Geometry check sheet. Reference: the model listing, model coordinates, mm. Face numbers are marked on the shaded views. A direction names the side the tool comes from. Round coordinates to 2 decimals unless told otherwise and drop trailing zeros. Order: outer loops, then holes, each group sorted by start corner. A loop starts at its lowest first (then second) coordinate and runs counter-clockwise, first axis right, second up.
(1) Thickness scan on L1, parallel to X at y = -6.5, z = 15.5; L2, parallel to Y at x = -9.5, z = 12; L3, parallel to Y at x = 0.5, z = 14. Record the ranges inside material, lowest first.
(2) Cross-section at C-C on x = 1.5. Enter the section's corners in (y, z).
(3) Set-up check for the marked faces 1, 2 and 3: record each of +Z, -Z, +X, -X, +Y, -Y from which the full face is reachable in a straight line by a thin tool's end or side.
(4) Draft check along X on the marked faces 4, 5, 6 and 7. Enter one of: pulls with the +X half, pulls with the -X half, needs draft (parallel to the pull), parting line crosses it, or undercut.
(5) Gauge pin test, flat ends, axial feed: P1, Ø6, axis at x = -6, y = -4, coming from the -Z side; P2, Ø4, axis at y = -6, z = 25.5, coming from the +X side; P3, Ø16, axis at x = 13, z = 12.5, coming from the +Y side (3 decimals); P4, Ø2, axis at y = 3, z = 18.5, coming from the +X side. Record the tip position at first contact, or that the pin passes through.
(6) Cross-section at B-B on y = -5.5. Enter the section's corners in (x, z).
(7) Cross-section at A-A on z = 15. Count the separate pieces of the cut face and the enclosed holes in it, and give its area (3 significant figures).
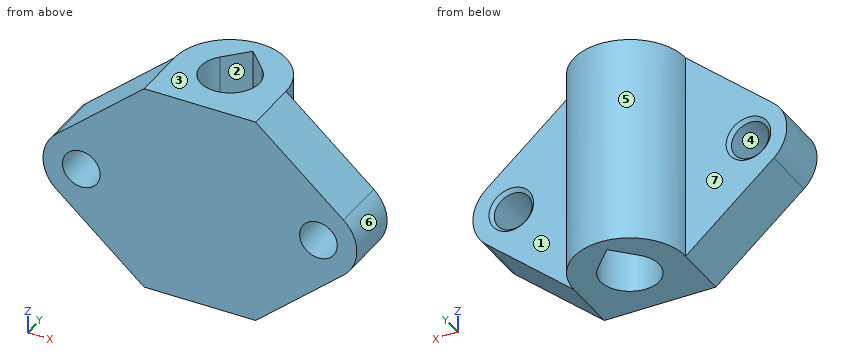
Solid Edge part; units mm, degrees
sketch "Sketch1" plane through (0, 0, 0) normal (0, 0, 1) x (1, 0, 0)
  circle A0 centre (0, 0) radius 4.1
  circle A1 centre (0, 0) radius 8
extrude "Protrusion1" add sketch "Sketch1" along normal blind 30
sketch "Sketch2" plane through (0, -8, 0) normal (0, -1, 0) x (1, 0, 0)
  arc A0 (-20.6265, 10.8649) -> (-20.548, 19.2026) centre (-17, 15) cw
  line L0 (-20.548, 19.2026) -> (-8, 30)
  line L1 (-8, 30) -> (8, 30)
  line L2 (8, 30) -> (20.5873, 19.1691)
  arc A1 (20.5873, 10.8309) -> (20.5873, 19.1691) centre (17, 15) ccw
  line L3 (8, 0) -> (20.5873, 10.8309)
  line L4 (8, 0) -> (-8, 0)
  line L5 (-20.6265, 10.8649) -> (-8, 0)
  circle A2 centre (-17, 15) radius 2.7
  circle A3 centre (17, 15) radius 2.7
extrude "Protrusion2" add sketch "Sketch2" against normal up to vertex (8 mm away)
sketch "Sketch3" plane through (0, 0, 30) normal (0, 0, 1) x (0, 1, 0)
  circle A0 centre (0, 0) radius 4.2
extrude "Cutout1" cut sketch "Sketch3" against normal through all
sketch "Sketch4" plane through (0, 0, 0) normal (0, 0, -1) x (-1, 0, 0)
  line L0 (0, 0) -> (3.0212, 2.9176)
  line L1 (3.0212, 2.9176) -> (0, 6.0461)
  line L2 (0, 6.0461) -> (-3.0212, 2.9176)
  line L3 (-3.0212, 2.9176) -> (0, 0)
extrude "Cutout2" cut sketch "Sketch4" against normal through all
chamfer "Chamfer_1" distance 0.5 angle 45 2 edges at (14.3, 0, 15) (-19.7, 0, 15)
Found:
1. L1: x = -22.48 to -19.65, -14.35 to 14.35, 19.65 to 22.48
1. L2: y = -8 to 0
1. L3: y = -8 to -4.17, 5.53 to 7.98
2. outline: (-8, 0) - (-3.92, 0) - (-3.92, 30) - (-8, 30) - close; (4.49, 0) - (7.86, 0) - (7.86, 30) - (4.49, 30) - close
3. face 1: +Z, -Z, +X, +Y
3. face 2: +Z, -Z
3. face 3: +Z, +X, -X, +Y, -Y
4. face 4: undercut
4. face 5: parting line crosses it
4. face 6: pulls with the +X half
4. face 7: needs draft
5. P1: stops at z = 0
5. P2: stops at x = 15.55
5. P3: stops at y = 6.245
5. P4: stops at x = 7.75
6. outline: (-20.63, 10.86) - (-8, 0) - (8, 0) - (20.59, 10.83) arc R5.5 ccw to (20.59, 19.17) - (8, 30) - (-8, 30) - (-20.55, 19.2) arc R5.5 ccw to start; hole circle Ø5.4 at (-17, 15); hole circle Ø5.4 at (17, 15)
7. separate pieces: 3
7. enclosed holes: 1
7. area: 314 mm2
